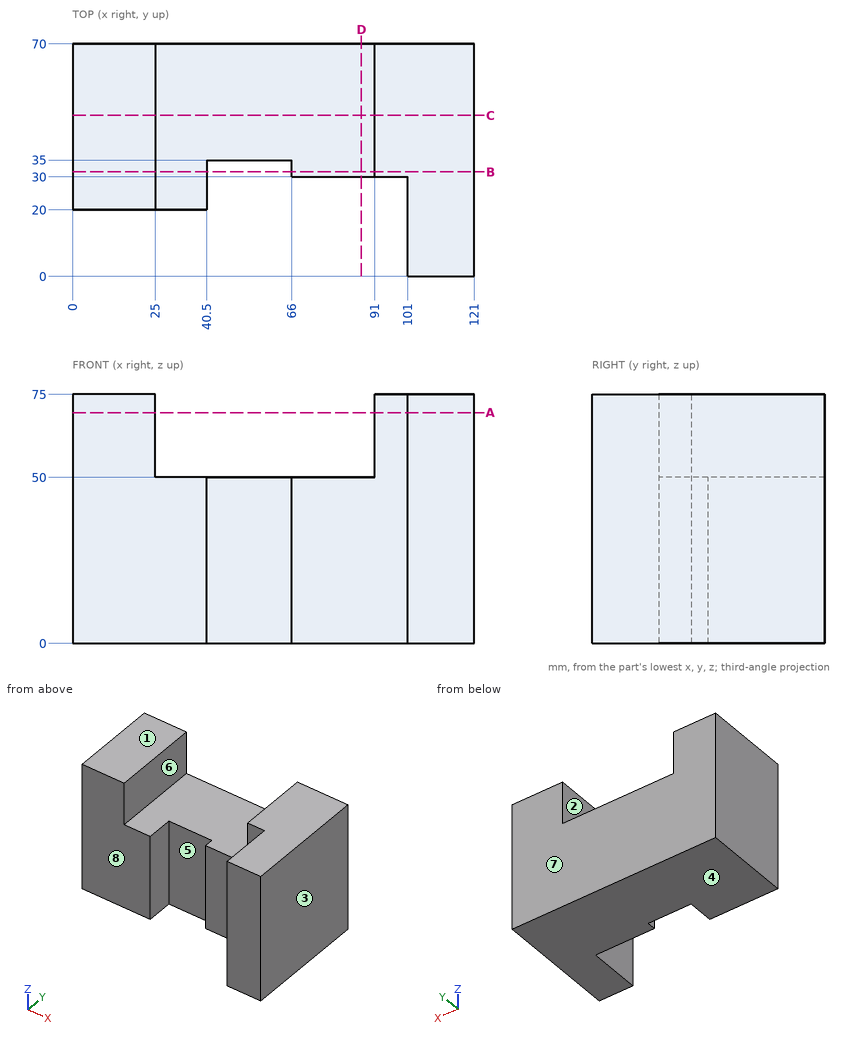
Source: three-view drawing plus pictorial views. Frame: mm from the lowest corner of the part. A direction names the side the tool comes from. Give positions to 0.01 mm unless a question says otherwise; leave off trailing zeros. Order: outer loops, then holes, each group sorted by start corner. A loop starts at its lowest first (then second) coordinate and runs counter-clockwise, first axis right, second up. Notation, with made-up numbers: (-35.5, 22) - (17.5, 22) arc R37 cw to (17.5, 59) - close; hole circle Ø10 at (69, -18). An arc over 180 degrees is marked (long way). Answer as a JSON object with one key per item and string values. Group by question number.
Q1. Set-up query: the marked faces 4, 5, 6, 7 and 8. Return all of +Z, -Z, +X, -X, +Y, -Y with unobstructed straight access to the full face (end or side cutting, diameter ignored); none if empty.
Q2. Cut plane D-D, the plane x = 87. Output: boundary loops of the cut face in (y, z).
Q3. Line query: probe 1 along X at (y, z) = (26.5, 27.5); probe 2 along X at (y, z) = (22, 65); probe 3 along Y at (x, z) = (53.5, 39). Output: solid intervals per line, ascending.
Q4. Mould query, pull axis X, two halves, no side actions, for the marked faces 1, 2 and 3. Classes: pulls with the +X half, pulls with the -X half, needs draft (parallel to the pull), parting line crosses it, or undercut.
Q5. Cut plane A-A, the plane z = 69.5. Output: boundary loops of the cut face in (x, y), then the cut area to 3 significant figures.
Q6. First-contact query: pin 1 Ø3 at (x, y) = (28, 58) entering from +Z; pin 2 Ø13 at (x, z) = (56, 26) entering from -Y; pin 3 Ø12 at (x, y) = (60.5, 21.5) entering from +Z. Flat tips, straight axial feed; report the tip coordinate or a pass-through.
Q7. Cut plane B-B, the plane y = 31.5. Output: boundary loops of the cut face in (x, z), then the cut area to 3 significant figures.
Q8. Cut plane C-C, the plane y = 48.5. Output: boundary loops of the cut face in (x, z).
Results:
{
 "1": {"face 4": "-Z, +X, -X, +Y, -Y", "face 5": "+Z, -Z, -Y", "face 6": "+Z, +Y, -Y", "face 7": "+Z, -Z, +X, -X, +Y", "face 8": "+Z, -Z, -X, -Y"},
 "2": {"outline": "(30, 0) - (70, 0) - (70, 50) - (30, 50) - close"},
 "3": {"probe 1": "0 to 40.5, 101 to 121", "probe 2": "0 to 25, 101 to 121", "probe 3": "35 to 70"},
 "4": {"face 1": "needs draft", "face 2": "undercut", "face 3": "pulls with the +X half"},
 "5": {"outline": "(0, 20) - (25, 20) - (25, 70) - (0, 70) - close; (91, 30) - (101, 30) - (101, 0) - (121, 0) - (121, 70) - (91, 70) - close", "area": "3,050 mm^2"},
 "6": {"pin 1": "z = 50", "pin 2": "y = 35", "pin 3": "through"},
 "7": {"outline": "(0, 0) - (40.5, 0) - (40.5, 50) - (25, 50) - (25, 75) - (0, 75) - close; (66, 0) - (121, 0) - (121, 75) - (91, 75) - (91, 50) - (66, 50) - close", "area": "6,150 mm^2"},
 "8": {"outline": "(0, 0) - (121, 0) - (121, 75) - (91, 75) - (91, 50) - (25, 50) - (25, 75) - (0, 75) - close"}
}
